```python
from build123d import *

# Parameters (mm, degrees)
SKETCH_1_W      = 77
SKETCH_1_H      = 72
SKETCH_1_R      = 1.05
EXTRUDE_1_DEPTH = 1.6
SKETCH_2_W      = 7
SKETCH_2_H      = 7
SKETCH_2_W_2    = 13.1
SKETCH_2_H_2    = 11.7
SKETCH_2_W_3    = 6
SKETCH_2_H_3    = 8
SKETCH_2_W_4    = 12.7
SKETCH_2_H_4    = 3.9
EXTRUDE_2_DEPTH = 2
SKETCH_3_W      = 7.6
SKETCH_3_H      = 8.9
EXTRUDE_3_DEPTH = 3
SKETCH_5_W      = 4.2
SKETCH_5_H      = 8.8
EXTRUDE_4_DEPTH = 5
SKETCH_6_W      = 27.7
SKETCH_6_H      = 3.9
EXTRUDE_5_DEPTH = 5


with BuildPart() as part:
    # 草图1 → 凸台-拉伸1 (new body)
    with BuildSketch(Plane(origin=(0, 0, 0), x_dir=(1, 0, 0), z_dir=(0, 1, 0))):
        with Locations((38.5, -36)):
            Rectangle(SKETCH_1_W, SKETCH_1_H)
        with Locations(Location((2, -2, 0), (0, 0, 270))):
            Circle(SKETCH_1_R, mode=Mode.SUBTRACT)
        with Locations(Location((2, -70, 0), (0, 0, 270))):
            Circle(SKETCH_1_R, mode=Mode.SUBTRACT)
        with Locations(Location((75, -2, 0), (0, 0, 270))):
            Circle(SKETCH_1_R, mode=Mode.SUBTRACT)
        with Locations(Location((75, -70, 0), (0, 0, 270))):
            Circle(SKETCH_1_R, mode=Mode.SUBTRACT)
    extrude(amount=EXTRUDE_1_DEPTH)

    # 草图2 → 凸台-拉伸2 (add)
    with BuildSketch(Plane(origin=(0, 1.6, 0), x_dir=(1, 0, 0), z_dir=(0, 1, 0))):
        with Locations((13.6, -20.5)):
            Rectangle(SKETCH_2_W, SKETCH_2_H)
        Polygon((44.1, -19.873088065), (27.836544033, -36.136544033), (44.1, -52.4), (60.363455967, -36.136544033), align=None)
        with Locations((15.85, -42.25)):
            Rectangle(SKETCH_2_W_2, SKETCH_2_H_2)
        with Locations((17, -53)):
            Rectangle(SKETCH_2_W_3, SKETCH_2_H_3)
        Polygon((65.835533906, -40.580909114), (55.15822151, -51.25822151), (62.3, -58.4), (72.977312396, -47.722687604), align=None)
        Polygon((60.864466094, -12.680909114), (53.722687604, -19.822687604), (64.4, -30.5), (71.54177849, -23.35822151), align=None)
        with Locations((67.85, -65.45)):
            Rectangle(SKETCH_2_W_4, SKETCH_2_H_4)
    extrude(amount=EXTRUDE_2_DEPTH)

    # 草图3 → 凸台-拉伸3 (add)
    with BuildSketch(Plane(origin=(0, 1.6, 0), x_dir=(1, 0, 0), z_dir=(0, 1, 0))):
        with Locations((73.2, -9.85)):
            Rectangle(SKETCH_3_W, SKETCH_3_H)
    extrude(amount=EXTRUDE_3_DEPTH)

    # 草图5 → 凸台-拉伸4 (add)
    with BuildSketch(Plane(origin=(0, 1.6, 0), x_dir=(1, 0, 0), z_dir=(0, 1, 0))):
        with Locations((2.4, -57.7)):
            Rectangle(SKETCH_5_W, SKETCH_5_H)
    extrude(amount=EXTRUDE_4_DEPTH)

    # 草图6 → 凸台-拉伸5 (add)
    with BuildSketch(Plane.XZ):
        with Locations((18.25, 66.95)):
            Rectangle(SKETCH_6_W, SKETCH_6_H)
        with Locations((47.13, 66.95)):
            Rectangle(SKETCH_6_W, SKETCH_6_H)
        with Locations((18.25, 5.05)):
            Rectangle(SKETCH_6_W, SKETCH_6_H)
        with Locations((47.13, 5.05)):
            Rectangle(SKETCH_6_W, SKETCH_6_H)
    extrude(amount=EXTRUDE_5_DEPTH)


solid = part.part
```
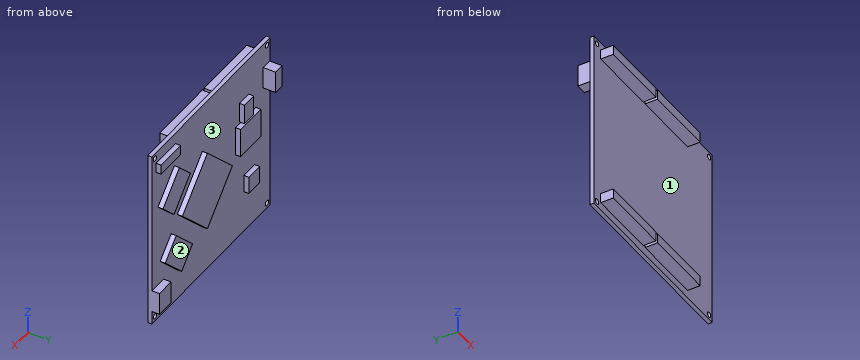
The listing builds one solid part. Answer for the finished solid, in the listing's coordinates (mm). Face numbers are marked on the shaded views. Coordinates: 2 decimals unless noted, no trailing zeros. Loops run counter-clockwise (first coordinate to the right, second up) from the corner with the lowest first, then second, coordinate; pieces in that order, holes last. Notation, with made-up numbers: (31, 33.5) - (63, 33.5) arc R20 ccw to (63, 39.5) - close; hole circle Ø11 at (-15, -11.5). An arc over 180 degrees is marked (long way). Use a Markdown table: item, result. Add a question column.
1) The part is cut by section A-A, the plane x = 2. Give the vertices of the cut face in (y, z).
2) The part is cut by section B-B, the plane y = -3. Give the vertices of the cut face in (x, z), and give its area (3 significant figures).
3) The mould has two halves that part along Z. Classify the marked faces 1, 2 and 3: released by +Z, released by -Z, zero draft, split by the parting line, or undercut.
4) Find the intervals of material crossed by line 1 (X direction, y = 0.75, z = 70); line 2 (Z direction, x = 27, y = -2.25); line 3 (Z direction, x = 75, y = 0.8), in increasing order.
5) The part is cut by section C-C, the plane z = 2. Give the vertices of the cut face in (x, y), and give its area (3 significant figures).
6) Given pin 1 (2 mm diameter, centred on x = 30, z = 29, fed in from -Y); pin 2 (1.3 mm diameter, centred on x = 2.5, y = 4.5, fed in from -Z); pin 3 (14.5 mm diameter, centred on x = 61, z = 45.5, fed in from +Y), each flat-ended and moving along its own axis, determine where each tip first touches the part or whether it passes through.
7) The part is cut by section D-D, the plane y = 2.5. State how many separate pieces and enclosed holes the cut face has, and give its area (3 significant figures).
Here are the results:
| question | item | result |
|---|---|---|
| 1 | outline | (0, 0) - (1.6, 0) - (1.6, 0.95) - (0, 0.95) - close; (0, 3.05) - (1.6, 3.05) - (1.6, 53.3) - (6.6, 53.3) - (6.6, 62.1) - (1.6, 62.1) - (1.6, 68.95) - (0, 68.95) - close; (0, 71.05) - (1.6, 71.05) - (1.6, 72) - (0, 72) - close |
| 2 | outline | (4.4, 3.1) - (32.1, 3.1) - (32.1, 7) - (4.4, 7) - close; (4.4, 65) - (32.1, 65) - (32.1, 68.9) - (4.4, 68.9) - close; (33.28, 3.1) - (60.98, 3.1) - (60.98, 7) - (33.28, 7) - close; (33.28, 65) - (60.98, 65) - (60.98, 68.9) - (33.28, 68.9) - close |
| 2 | area | 432 mm^2 |
| 3 | face 1 | undercut |
| 3 | face 2 | zero draft |
| 3 | face 3 | undercut |
| 4 | line 1 | x = 0 to 0.95, 3.05 to 73.95, 76.05 to 77 |
| 4 | line 2 | z = 3.1 to 7, 65 to 68.9 |
| 4 | line 3 | z = 0 to 0.95, 3.05 to 68.95, 71.05 to 72 |
| 5 | outline | (0, 0) - (0.95, 0) - (0.95, 1.6) - (0, 1.6) - close; (3.05, 0) - (73.95, 0) - (73.95, 1.6) - (3.05, 1.6) - close; (76.05, 0) - (77, 0) - (77, 1.6) - (76.05, 1.6) - close |
| 5 | area | 116 mm^2 |
| 6 | pin 1 | stops at y = 0 |
| 6 | pin 2 | stops at z = 53.3 |
| 6 | pin 3 | stops at y = 3.6 |
| 7 | separate pieces | 9 |
| 7 | enclosed holes | 0 |
| 7 | area | 1,240 mm^2 |
